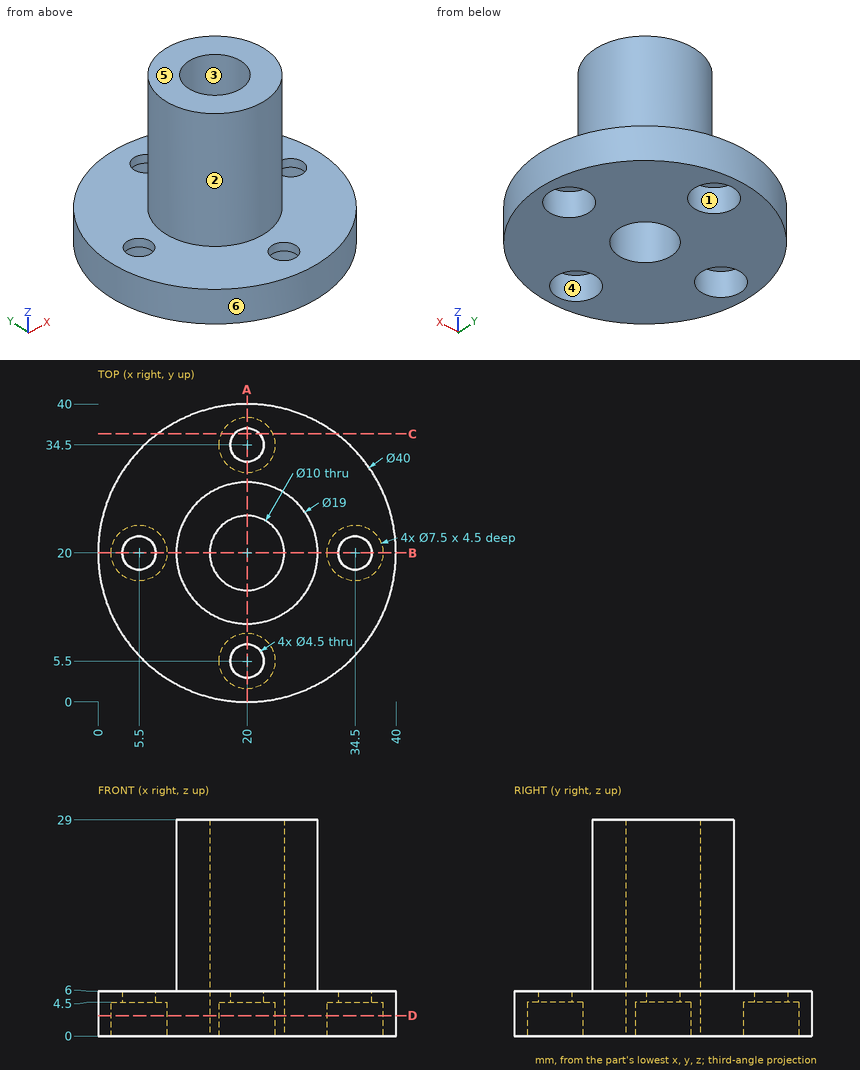
Geometry check sheet. Reference: drawing and pictorial views, mm from the part's lowest x, y, z. A direction names the side the tool comes from. Give positions to 0.01 mm unless a question says otherwise; leave off trailing zeros. Order: outer loops, then holes, each group sorted by start corner. A loop starts at its lowest first (then second) coordinate and runs counter-clockwise, first axis right, second up. Notation, with made-up numbers: (-17.75, 78.25) - (-0.75, 78.25) arc R14 cw to (-0.75, 103.25) - close; hole circle Ø10 at (74.25, 48.25). An arc over 180 degrees is marked (long way). Use one line per item in the form item = value.
1) Depth check by flat-ended pin: pin 1 Ø8 at (x, y) = (4.5, 34) entering from -Z; pin 2 Ø10 at (y, z) = (33.5, 24.5) entering from +X; pin 3 Ø2.5 at (x, y) = (34.5, 20) entering from -Z; pin 4 Ø6 at (x, y) = (5.5, 20) entering from -Z. Enter the tip coordinate at first touch or a pass-through.
Working result:
pin_1 = 0
pin_2 = 24.24
pin_3 = through
pin_4 = 4.5
2) Draft check along X on the marked faces 4, 5 and 6. Enter one of: released by +X, released by -X, zero draft, split by the parting line, or undercut.
Working result:
face_4 = undercut
face_5 = zero draft
face_6 = split by the parting line
3) Material ranges on probe 1 along Y at (x, z) = (20, 5.45); probe 2 along Y at (x, z) = (20, 2.25); probe 3 along Y at (x, z) = (20, 16.25), recorded low to high. Write a range as from..to.
Working result:
probe_1 = 0..3.25, 7.75..15, 25..32.25, 36.75..40
probe_2 = 0..1.75, 9.25..15, 25..30.75, 38.25..40
probe_3 = 10.5..15, 25..29.5
4) Sectioned sample at C-C (y = 36). Record the boundary of the cut face in (x, z).
Working result:
outline = (8, 0) - (16.56, 0) - (16.56, 4.5) - (18.32, 4.5) - (18.32, 6) - (8, 6) - close; (21.68, 4.5) - (23.44, 4.5) - (23.44, 0) - (32, 0) - (32, 6) - (21.68, 6) - close
5) Sectioned sample at A-A (x = 20). Record the boundary of the cut face in (y, z), and give its area (3 significant figures).
Working result:
outline = (0, 0) - (1.75, 0) - (1.75, 4.5) - (3.25, 4.5) - (3.25, 6) - (0, 6) - close; (7.75, 4.5) - (9.25, 4.5) - (9.25, 0) - (15, 0) - (15, 29) - (10.5, 29) - (10.5, 6) - (7.75, 6) - close; (25, 0) - (30.75, 0) - (30.75, 4.5) - (32.25, 4.5) - (32.25, 6) - (29.5, 6) - (29.5, 29) - (25, 29) - close; (36.75, 4.5) - (38.25, 4.5) - (38.25, 0) - (40, 0) - (40, 6) - (36.75, 6) - close
area = 306 mm^2
6) Sectioned sample at D-D (z = 2.75). Record the boundary of the cut face in (x, y), and give its area (3 significant figures).
Working result:
outline = circle Ø40 at (20, 20); hole circle Ø7.5 at (5.5, 20); hole circle Ø10 at (20, 20); hole circle Ø7.5 at (20, 5.5); hole circle Ø7.5 at (20, 34.5); hole circle Ø7.5 at (34.5, 20)
area = 1,000 mm^2
7) Access from +Z, -Z, +X, -X, +Y, -Y to the whole of each face (thin tool, end or side, straight path). Record for the marked faces 1, 2 and 3.
Working result:
face_1 = -Z
face_2 = +Z
face_3 = +Z, -Z
